The drawing under review shows one solid part. Ordinate dimensions are in mm from its lowest x, y, z. Round coordinates to 2 decimals unless told otherwise and drop trailing zeros. Order: outer loops, then holes, each group sorted by start corner. A loop starts at its lowest first (then second) coordinate and runs counter-clockwise, first axis right, second up. Notation, with made-up numbers: M 17.25,-39 L 43.25,-39 A23 cw 43.25,-1 Z; hole C 40.25,1.25 d5. An arc over 180 degrees is marked long. Answer as a JSON object with one key per item and string values. Group by question number.
1) Consider section C-C, the plane x = 2.5. Write out the cut boundary in (y, z).
2) Insertion check: pin 1 Ø1 at (y, z) = (5, 22) entering from -X; pin 2 Ø1.5 at (y, z) = (1, 9) entering from +X; pin 3 Ø2.5 at (x, z) = (3.175, 3.81) entering from +Y. Each pin has a flat end and moves straight along its axis. Give the tip position at first contact, or say it passes through.
3) To check wall thickness, follow line 1 (Y direction, x = 3, z = 40.5) (1 decimal); line 2 (X direction, y = 3.05, z = 17); line 3 (Y direction, x = 4.75, z = 12.5). State the ranges of each line that lie inside material, in increasing order.
4) Consider section A-A, the plane y = 2.8. Write out the cut boundary in (x, z).
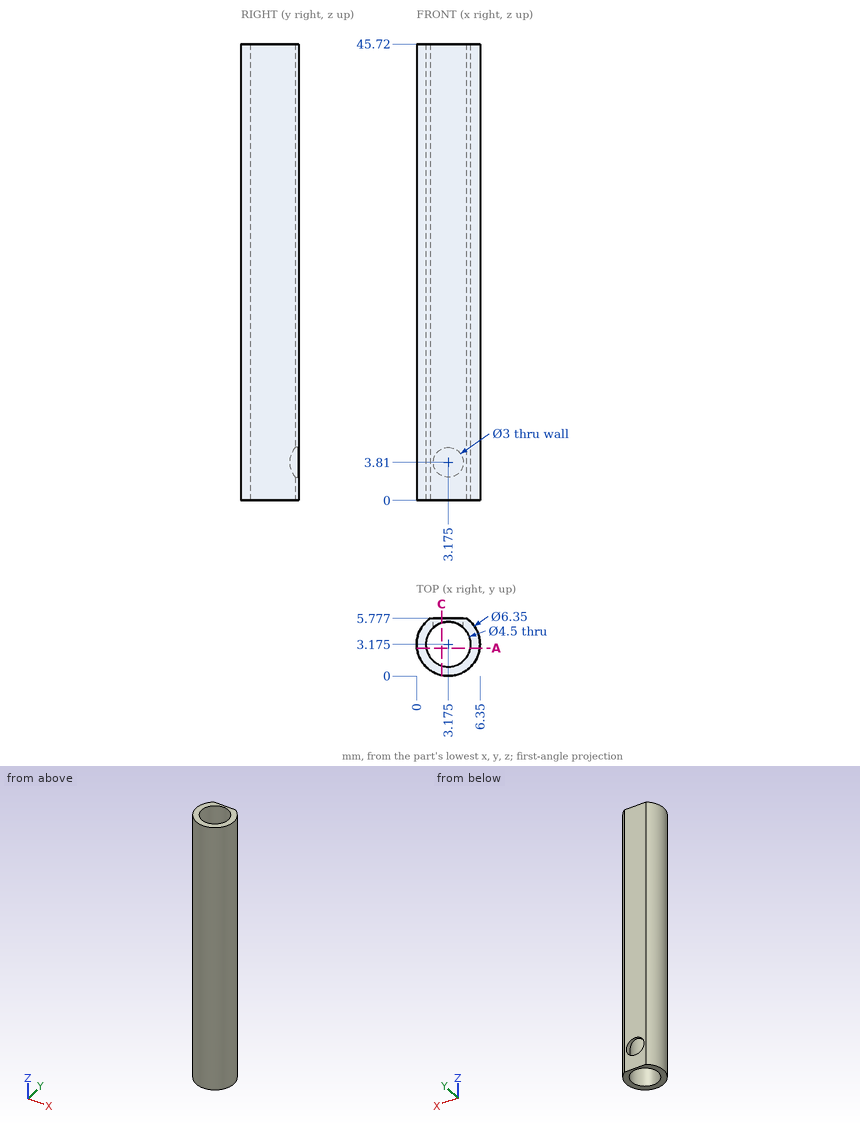
Results list:
{
 "1": {"outline": "M 0.07,0 L 1.03,0 L 1.03,45.72 L 0.07,45.72 Z; M 5.32,0 L 5.78,0 L 5.78,2.47 L 5.32,2.47 Z; M 5.32,5.15 L 5.78,5.15 L 5.78,45.72 L 5.32,45.72 Z"},
 "2": {"pin 1": "x = 0.29", "pin 2": "x = 6.01", "pin 3": "y = 1.3"},
 "3": {"line 1": "0 to 0.9, 5.4 to 5.8", "line 2": "0 to 0.93, 5.42 to 6.35", "line 3": "0.42 to 1.57, 4.78 to 5.78"},
 "4": {"outline": "M 0.02,0 L 0.96,0 L 0.96,45.72 L 0.02,45.72 Z; M 5.39,0 L 6.33,0 L 6.33,45.72 L 5.39,45.72 Z"}
}
